Geometry check sheet. Reference: the model listing, model coordinates, mm. A direction names the side the tool comes from. Give positions to 0.01 mm unless a question says otherwise; leave off trailing zeros. Order: outer loops, then holes, each group sorted by start corner. A loop starts at its lowest first (then second) coordinate and runs counter-clockwise, first axis right, second up. Notation, with made-up numbers: M 46,-33 L 69,-33 A5 cw 69,-24 Z; hole C 31.5,-29 d1. An arc over 180 degrees is marked long. Answer as CSV lines item,"result". Start each with the question number.
Q1. Thickness scan on line 1 (Y direction, x = -10, z = -9.65); line 2 (Y direction, x = -96, z = -27); line 3 (X direction, y = 46.5, z = -6). Record the ranges inside material, lowest first.
Q2. Section check B-B, the plane z = -27. Record the boundary of the cut face in (x, y).
Q3. Section check C-C, the plane y = 2. Record the boundary of the cut face in (x, z), then the cut area to 3 significant figures.
Q4. Go/stop test with flat-tipped pins: pin 1 (11.5 mm diameter, centred on x = -60, y = -49, fed in from +Z); pin 2 (1 mm diameter, centred on x = -58.5, y = 4.5, fed in from -Z); pin 3 (7.5 mm diameter, centred on x = -94.5, z = -15, fed in from -Y). Record where each tip stops, or that it passes through.
Q5. Section check D-D, the plane y = -49. Record the boundary of the cut face in (x, z), then the cut area to 3 significant figures.
Q6. Mould release check, pull along X, two halves, no side actions. Record for faces 1 (the flat face through (-102, 1, -20)), 2 (the cylindrical face through (-61.352, 44.708, -10.521)), 3 (the cylindrical face through (-94.62, 23.85, -27.55)): +X half, -X half, draft (parallel to the pull), parting line (faces both ways), or undercut.
Q7. Set-up check for faces 4 (the cylindrical face through (-8.648, -44.708, -10.521)), 5 (the flat face through (-89, 1, -25)), 6 (the flat face through (-5, 49, -9)): record each of +Z, -Z, +X, -X, +Y, -Y from which the full face is reachable in a straight line by a thin tool's end or side.
Q8. Section check A-A, the plane x = -60. Record the boundary of the cut face in (y, z), then the cut area to 3 significant figures.
Autodesk Inventor part; units mm, degrees
ref_plane "YZ Plane" through (0, 0, 0) normal (1, 0, 0) x (0, 1, 0)
ref_plane "XZ Plane" through (0, 0, 0) normal (0, 1, 0) x (-1, 0, 0)
ref_plane "XY Plane" through (0, 0, 0) normal (0, 0, 1) x (1, 0, 0)
sketch "Эскиз1" plane through (0, 0, 0) normal (0, 0, 1) x (1, 0, 0)
  line L0 (0, 0) -> (0, 58)
  line L1 (0, 58) -> (-65, 58)
  line L2 (-65, 58) -> (-76.547, 38)
  line L3 (-76.547, 38) -> (-102, 38)
  line L4 (-102, 38) -> (-102, 0)
  line L5 (-102, 0) -> (0, 0)
  line L6 (-89, 38) -> (-89, 0)
  point P0 (-60, 49)
  point P1 (-10, 49)
  dimension "d0" = 116
  dimension "d1" = 76
  dimension "d2" = 60
  dimension "d3" = 65
  dimension "d4" = 102
  dimension "d5" = 13
  dimension "d6" = 50
  dimension "d7" = 10
  dimension "d8" = 98
extrude "Выдавливание1" add sketch "Эскиз1" against normal blind 12 contours L5 L6 L3 L2 L1 L0
extrude "Выдавливание2" add sketch "Эскиз1" against normal blind 38 contours L5 L4 L3 L6
hole "Отверстие1" at (-60, 49, 0) at (-10, 49, 0) direction (0, 0, -1) diameter 9 end through all counterbore diameter 14 counterbore depth 9
hole "Отверстие2" at (-102, 28, -27) direction (1, 0, 0) diameter 8.376 end through all
chamfer "Фаска1" distance 1.6 angle 45 1 edges at (-102, 28, -31.188)
chamfer "Фаска2" distance 3 angle 45 1 edges at (-102, 19, 0)
chamfer "Фаска3" distance 2 angle 45 1 edges at (0, 58, -6)
mirror "Зеркальное отражение1" about plane through (0, 0, 0) normal (0, -1, 0)
properties part number "Крышка 6"
Answer block:
1,line 1,"y = -58 to -53.5, -44.5 to 44.5, 53.5 to 58"
1,line 2,"y = -38 to -32.19, -23.81 to 23.81, 32.19 to 38"
1,line 3,"x = -71.64 to -66.54, -53.46 to -16.54, -3.46 to 0"
2,outline,"M -102,-38 L -89,-38 L -89,-32.19 L -100.4,-32.19 L -102,-33.79 Z; M -102,-22.21 L -100.4,-23.81 L -89,-23.81 L -89,23.81 L -100.4,23.81 L -102,22.21 Z; M -102,33.79 L -100.4,32.19 L -89,32.19 L -89,38 L -102,38 Z"
3,outline,"M -102,-38 L -89,-38 L -89,-12 L 0,-12 L 0,0 L -99,0 L -102,-3 Z"
3,area,"1,560 mm2"
4,pin 1,"stops at z = -9"
4,pin 2,"stops at z = -12"
4,pin 3,"stops at y = -38"
5,outline,"M -70.2,-12 L -64.5,-12 L -64.5,-9 L -67,-9 L -67,0 L -70.2,0 Z; M -55.5,-12 L -14.5,-12 L -14.5,-9 L -17,-9 L -17,0 L -53,0 L -53,-9 L -55.5,-9 Z; M -5.5,-12 L 0,-12 L 0,0 L -3,0 L -3,-9 L -5.5,-9 Z"
5,area,"536 mm2"
6,face 1,"-X half"
6,face 2,"undercut"
6,face 3,"draft"
7,face 4,"+Z, -Z"
7,face 5,"-Z, +X, +Y, -Y"
7,face 6,"+Z"
8,outline,"M -58,-12 L -53.5,-12 L -53.5,-9 L -56,-9 L -56,0 L -58,0 Z; M -44.5,-12 L 44.5,-12 L 44.5,-9 L 42,-9 L 42,0 L -42,0 L -42,-9 L -44.5,-9 Z; M 53.5,-12 L 58,-12 L 58,0 L 56,0 L 56,-9 L 53.5,-9 Z"
8,area,"1,090 mm2"
